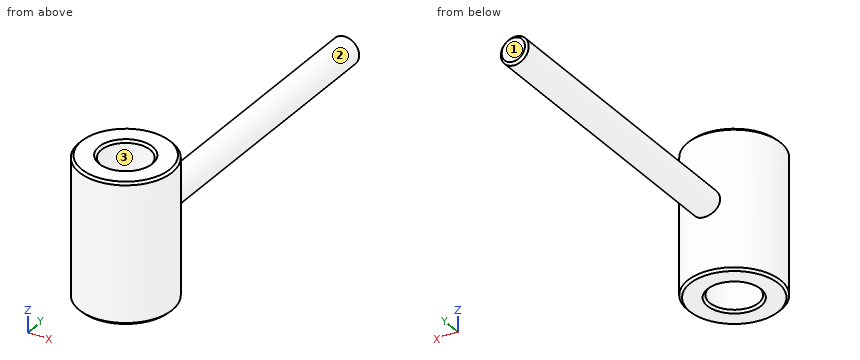
```python
from build123d import *

# Parameters (mm, degrees)
F0_R     = 20
F1_DEPTH = 30
F3_D     = 21
F5_R     = 6
F7_SIZE  = 1


with BuildPart() as f1:
    # F0 (on Top) → F1 (new body, symmetric)
    with BuildSketch(Plane.XY):
        Circle(F0_R)
    extrude(amount=F1_DEPTH, both=True)

    # F3 (through all)
    with Locations(Plane.XY.offset(30)):
        with Locations((0, 0)):
            Hole(F3_D / 2)

    # F5 (on offset) → F6 (join, up to the next surface of F1)
    with BuildSketch(Plane.XZ.offset(-150)):
        Circle(F5_R)
    extrude(until=Until.NEXT)

    # F7
    f7_edges = [f1.edges().sort_by_distance(p)[0] for p in [
        (-6, 150, 0),
        (-20, 0, 30),
        (-20, 0, -30),
        (-10.5, 0, 30),
        (-10.5, 0, -30),
    ]]
    chamfer(f7_edges, length=F7_SIZE)


solid = f1.part
```
Source: CAD feature listing. Evaluate the final solid. Frame: model axes, mm. Face numbers are marked on the shaded views. Round coordinates to 2 decimals unless told otherwise and drop trailing zeros. Loops run counter-clockwise (first coordinate to the right, second up) from the corner with the lowest first, then second, coordinate; pieces in that order, holes last.
1. Section query A-A on x = 0. Output: boundary loops of the cut face in (y, z).
2. Section query C-C on y = 0. Output: boundary loops of the cut face in (x, z).
3. Mould query, pull axis Y, two halves, no side actions, for the marked faces 1, 2 and 3. Classes: released by +Y, released by -Y, zero draft, split by the parting line, or undercut.
4. Ray query, L1, parallel to Y at x = 0, z = -13; L2, parallel to Y at x = 0, z = -3; L3, parallel to X at y = 125.5, z = 0.5. Return the intervals inside material, ascending.
5. Section query D-D on y = 37.5. Output: boundary loops of the cut face in (x, z), and give its area (3 significant figures).
6. Section query B-B on z = 0. Output: boundary loops of the cut face in (x, y).
7. Contact query for flat-ended pins moving along their axis: pin 1 (2 mm diameter, centred on y = 107.5, z = 5.5, fed in from -X); pin 2 (4 mm diameter, centred on y = 3, z = 3.5, fed in from -X) (3 decimals); pin 3 (4 mm diameter, centred on x = -8.5, z = -5.5, fed in from +Y). Output: stop coordinate, or through.
Answers below:
1. outline: (-20, -29) - (-19, -30) - (-11.5, -30) - (-10.5, -29) - (-10.5, 29) - (-11.5, 30) - (-19, 30) - (-20, 29) - close; (10.5, -29) - (11.5, -30) - (19, -30) - (20, -29) - (20, -6) - (149, -6) - (150, -5) - (150, 5) - (149, 6) - (20, 6) - (20, 29) - (19, 30) - (11.5, 30) - (10.5, 29) - close
2. outline: (-20, -29) - (-19, -30) - (-11.5, -30) - (-10.5, -29) - (-10.5, 29) - (-11.5, 30) - (-19, 30) - (-20, 29) - close; (10.5, -29) - (11.5, -30) - (19, -30) - (20, -29) - (20, 29) - (19, 30) - (11.5, 30) - (10.5, 29) - close
3. face 1: released by +Y
3. face 2: zero draft
3. face 3: undercut
4. L1: y = -20 to -10.5, 10.5 to 20
4. L2: y = -20 to -10.5, 10.5 to 150
4. L3: x = -5.98 to 5.98
5. outline: circle Ø12 at (0, 0)
5. area: 113 mm2
6. outline: (-6, 19.08) arc R20 ccw (long way) to (6, 19.08) - (6, 149) - (5, 150) - (-5, 150) - (-6, 149) - close; hole circle Ø21 at (0, 0)
7. pin 1: stops at x = -3.97
7. pin 2: stops at x = -19.975
7. pin 3: stops at y = 18.91
